from build123d import *

# Parameters (mm, degrees)
F0_W        = 16.002
F0_H        = 60.96
F0_R        = 1.27
F0_W_2      = 1.905
F1_DEPTH    = 1.524
F2_T1_DEPTH = 72.5997422652
F3_W        = 15.748
F3_H        = 0.254
F4_DEPTH    = 25.4
F5_R        = 0.635
F6_R        = 0.254


# Not quite as in the source:
# - a fillet or chamfer that OpenCascade refuses, or shapes differently, is made with other operations: its cross-section is extruded or revolved along the edge and cut away or added


with BuildPart() as f1:
    # F0 (on Top) → F1 (new body)
    with BuildSketch(Plane.XY):
        Rectangle(F0_W, F0_H)
        with Locations((0, -27.94)):
            Circle(F0_R, mode=Mode.SUBTRACT)
        with Locations((0, 27.94)):
            Circle(F0_R, mode=Mode.SUBTRACT)
        with Locations((-8.9535, 0)):
            Rectangle(F0_W_2, F0_H)
        with Locations((8.9535, 0)):
            Rectangle(F0_W_2, F0_H)
    extrude(amount=F1_DEPTH)

    # F2: fillet of radius 2.54 on 2 edges, made by hand

    # F2_s2 → F2_t1 (cut)
    with BuildSketch(Plane.XZ.offset(-36.2998711326)):
        with BuildLine():
            ThreePointArc((-9.906, 0), (-8.969266843, 1.1091164674), (-7.578051547, 1.524))
            Line((-7.578051547, 1.524), (-9.906, 1.524))
            Line((-9.906, 1.524), (-9.906, 0))
        make_face()
        with BuildLine():
            ThreePointArc((9.906, 0), (8.969266843, 1.1091164674), (7.578051547, 1.524))
            Line((7.578051547, 1.524), (9.906, 1.524))
            Line((9.906, 1.524), (9.906, 0))
        make_face()
    extrude(amount=F2_T1_DEPTH, mode=Mode.SUBTRACT)

    # F3 (on Top) → F4 (cut)
    with BuildSketch(Plane.XY):
        with Locations((0, 30.353)):
            Rectangle(F3_W, F3_H)
        Polygon((11.6183462764, 30.48), (7.874, 30.48), (7.874, 30.226), (7.874, -30.226), (7.874, -30.48), (11.6183462764, -30.48), align=None)
        Polygon((-7.874, 30.226), (-7.874, 30.48), (-11.6183462764, 30.48), (-11.6183462764, -30.48), (-7.874, -30.48), (-7.874, -30.226), align=None)
        with Locations((0, -30.353)):
            Rectangle(F3_W, F3_H)
    extrude(amount=F4_DEPTH, mode=Mode.SUBTRACT)

    # F5
    f5_edges = [f1.edges().sort_by_distance(p)[0] for p in [
        (-7.874, 30.226, 0.75335),
        (7.874, 30.226, 0.75335),
        (-7.874, -30.226, 0.75335),
        (7.874, -30.226, 0.75335),
        (0, -30.226, 0),
        (-7.874, 0, 0),
        (0, 30.226, 0),
        (7.874, 0, 0),
    ]]
    fillet(f5_edges, radius=F5_R)

    # F6
    f6_edges = [f1.edges().sort_by_distance(p)[0] for p in [
        (0, -30.226, 1.524),
        (-1.27, -27.94, 1.524),
        (-1.27, 27.94, 1.524),
        (7.874, 0, 1.5067),
        (-7.874, 0, 1.5067),
        (0, 30.226, 1.524),
        (7.415478, 30.200984, 1.524),
        (7.415478, -30.200984, 1.524),
        (-7.415478, 30.200984, 1.524),
        (-7.415478, -30.200984, 1.524),
        (7.798093, -29.892064, 1.514451),
        (-7.798115, -29.892025, 1.514449),
        (7.798115, 29.892025, 1.514449),
        (-7.798115, 29.892025, 1.514449),
    ]]
    fillet(f6_edges, radius=F6_R)


solid = f1.part
Input: part model. Units: mm. Frame: model coordinates. Coordinates: 2 decimals unless noted, no trailing zeros. Loops run counter-clockwise (first coordinate to the right, second up) from the corner with the lowest first, then second, coordinate; pieces in that order, holes last. Notation, with made-up numbers: (89.25, 24) - (127.25, 24) arc R24 cw to (127.25, 37) - close; hole circle Ø1 at (62.5, 84.5). An arc over 180 degrees is marked (long way). Answer in a Markdown table with one row per item. Add a question column.
Item 1: Line query: line 1 along Y through (x, z) = (0, 1); line 2 along X through (y, z) = (-2, 1.45); line 3 along X through (y, z) = (-24, 1.3). Output: solid intervals per line, ascending. Write a range as [from, to].
Item 2: Section query B-B on x = 0. Return the cut outline in (y, z) (3 decimals), then the cut area to 3 significant figures.
Item 3: Mould query, pull axis Y, two halves, no side actions, for faces 1 (the flat face through (0, 0, 1.524)), 2 (the cylindrical face through (0.7, 29, 0.6)), 3 (the cylindrical face through (-0.17, -26.68, 0.63)). Classes: released by +Y, released by -Y, zero draft, split by the parting line, or undercut.
Item 4: Section query A-A on y = -27.94. Return the cut outline in (x, z) (3 decimals).
Item 5: Contact query for flat-ended pins moving along their axis: P1, Ø2, axis at x = 0, y = 27.94, coming from the +Z side; P2, Ø1, axis at x = -3, y = -12.5, coming from the -Z side. Output: stop coordinate, or through.
Item 6: Section query C-C on z = 0.25. Return the cut outline in (x, y), then the cut area to 3 significant figures.
Recorded:
| question | item | result |
|---|---|---|
| 1 | line 1 | [-30.23, -29.21], [-26.67, 26.67], [29.21, 30.23] |
| 1 | line 2 | [-7.8, 7.8] |
| 1 | line 3 | [-7.87, 7.87] |
| 2 | outline | (-30.226, 0.635) arc R0.635 ccw to (-29.591, 0) - (-29.21, 0) - (-29.21, 1.27) arc R0.254 ccw to (-29.464, 1.524) - (-29.972, 1.524) arc R0.254 ccw to (-30.226, 1.27) - close; (-26.67, 0) - (26.67, 0) - (26.67, 1.27) arc R0.254 ccw to (26.416, 1.524) - (-26.416, 1.524) arc R0.254 ccw to (-26.67, 1.27) - close; (29.21, 0) - (29.591, 0) arc R0.635 ccw to (30.226, 0.635) - (30.226, 1.27) arc R0.254 ccw to (29.972, 1.524) - (29.464, 1.524) arc R0.254 ccw to (29.21, 1.27) - close |
| 2 | area | 84.1 mm^2 |
| 3 | face 1 | zero draft |
| 3 | face 2 | undercut |
| 3 | face 3 | undercut |
| 4 | outline | (-7.874, 0.635) arc R0.635 ccw to (-7.239, 0) - (-1.27, 0) - (-1.27, 1.27) arc R0.254 ccw to (-1.524, 1.524) - (-7.578, 1.524) arc R2.54 ccw to (-7.625, 1.524) arc R0.254 ccw to (-7.874, 1.27) - close; (1.27, 0) - (7.239, 0) arc R0.635 ccw to (7.874, 0.635) - (7.874, 1.27) arc R0.254 ccw to (7.625, 1.524) arc R2.54 ccw to (7.578, 1.524) - (1.524, 1.524) arc R0.254 ccw to (1.27, 1.27) - close |
| 5 | P1 | through |
| 5 | P2 | z = 0 |
| 6 | outline | (-7.74, -29.59) arc R0.5 ccw to (-7.24, -30.1) - (7.24, -30.1) arc R0.5 ccw to (7.74, -29.59) - (7.74, 29.59) arc R0.5 ccw to (7.24, 30.1) - (-7.24, 30.1) arc R0.5 ccw to (-7.74, 29.59) - close; hole circle Ø2.54 at (0, -27.94); hole circle Ø2.54 at (0, 27.94) |
| 6 | area | 922 mm^2 |
